Check sheet for the modelled part. Datum: model origin and axes. Units: mm. A direction names the side the tool comes from. Give positions to 0.01 mm unless a question says otherwise; leave off trailing zeros. Order: outer loops, then holes, each group sorted by start corner. A loop starts at its lowest first (then second) coordinate and runs counter-clockwise, first axis right, second up.
from build123d import *

# Parameters (mm, degrees)
F1_DEPTH = 3.5
F0_W     = 4
F0_H     = 15
F2_DEPTH = 1


with BuildPart() as f1:
    # F0 (on Front) → F1 (new body, symmetric)
    with BuildSketch(Plane.XZ):
        Polygon((80, -3), (80, 3), (-80, 3), (-80, -3), (-73, -3), (73, -3), align=None)
        Polygon((73, -9), (73, -3), (-73, -3), (-73, -9), (-69.25, -9), (-65.25, -9), (-60.25, -9), (-56.25, -9), (-51.25, -9), (-47.25, -9), (-42.25, -9), (-38.25, -9), (-33.25, -9), (-29.25, -9), (-24.25, -9), (-20.25, -9), (-15.25, -9), (-11.25, -9), (-6.25, -9), (-2.25, -9), (2.75, -9), (6.75, -9), (11.75, -9), (15.75, -9), (20.75, -9), (24.75, -9), (29.75, -9), (33.75, -9), (38.75, -9), (42.75, -9), (47.75, -9), (51.75, -9), (56.75, -9), (60.75, -9), (65.75, -9), (69.75, -9), align=None)
    extrude(amount=F1_DEPTH, both=True)

    # F0 (on Front) → F2 (join, symmetric)
    with BuildSketch(Plane.XZ):
        with Locations((67.75, -16.5)):
            Rectangle(F0_W, F0_H)
        with Locations((58.75, -16.5)):
            Rectangle(F0_W, F0_H)
        with Locations((49.75, -16.5)):
            Rectangle(F0_W, F0_H)
        with Locations((40.75, -16.5)):
            Rectangle(F0_W, F0_H)
        with Locations((31.75, -16.5)):
            Rectangle(F0_W, F0_H)
        with Locations((22.75, -16.5)):
            Rectangle(F0_W, F0_H)
        with Locations((13.75, -16.5)):
            Rectangle(F0_W, F0_H)
        with Locations((4.75, -16.5)):
            Rectangle(F0_W, F0_H)
        with Locations((-4.25, -16.5)):
            Rectangle(F0_W, F0_H)
        with Locations((-13.25, -16.5)):
            Rectangle(F0_W, F0_H)
        with Locations((-22.25, -16.5)):
            Rectangle(F0_W, F0_H)
        with Locations((-31.25, -16.5)):
            Rectangle(F0_W, F0_H)
        with Locations((-40.25, -16.5)):
            Rectangle(F0_W, F0_H)
        with Locations((-49.25, -16.5)):
            Rectangle(F0_W, F0_H)
        with Locations((-58.25, -16.5)):
            Rectangle(F0_W, F0_H)
        with Locations((-67.25, -16.5)):
            Rectangle(F0_W, F0_H)
    extrude(amount=F2_DEPTH, both=True)


solid = f1.part
1) Section check C-C, the plane z = -6. Record the cut outline in (x, y), then the cut area to 3 significant figures.
Recorded:
outline: (-73, -3.5) - (73, -3.5) - (73, 3.5) - (-73, 3.5) - close
area: 1,020 mm2
2) Draft check along X on faces 5 (the face through (-80, 0, 0)), 6 (the face through (-1, 0, -9)), 7 (the face through (-67, -1, -16)), 8 (the face through (73, 0, -6)). Enter one of: +X half, -X half, draft (parallel to the pull), parting line (faces both ways), or undercut.
Recorded:
face 5: -X half
face 6: undercut
face 7: draft
face 8: +X half
3) Depth check by flat-ended pin: pin 1 Ø8 at (x, z) = (-39.5, -21) entering from -Y; pin 2 Ø1 at (y, z) = (0.5, -15.5) entering from -X; pin 3 Ø4.5 at (x, z) = (4, -14) entering from +Y. Enter the tip coordinate at first touch or a pass-through.
Recorded:
pin 1: stops at y = -1
pin 2: stops at x = -69.25
pin 3: stops at y = 1
4) Section check A-A, the plane z = -22.5. State how many separate pieces and enclosed holes the cut face has, then the cut area to 3 significant figures.
Recorded:
separate pieces: 16
enclosed holes: 0
area: 128 mm2
5) Material ranges on L1, parallel to Y at x = -59, z = -21.5; L2, parallel to Z at x = -51, y = -1.25; L3, parallel to X at y = 2.5, z = -8, recorded low to high.
Recorded:
L1: y = -1 to 1
L2: z = -9 to 3
L3: x = -73 to 73
6) Set-up check for faces 1 (the face through (-1, 3.5, -3)), 2 (the face through (-77, 0, -3)), 3 (the face through (32, 1, -16)), 4 (the face through (50, -1, -16)): record each of +Z, -Z, +X, -X, +Y, -Y from which the full face is reachable in a straight line by a thin tool's end or side.
Recorded:
face 1: +Z, -Z, +X, -X, +Y
face 2: -Z, -X, +Y, -Y
face 3: -Z, +X, -X, +Y
face 4: -Z, +X, -X, -Y
7) Section check B-B, the plane x = 19. Record the cut outline in (y, z).
Recorded:
outline: (-3.5, -9) - (3.5, -9) - (3.5, 3) - (-3.5, 3) - close
